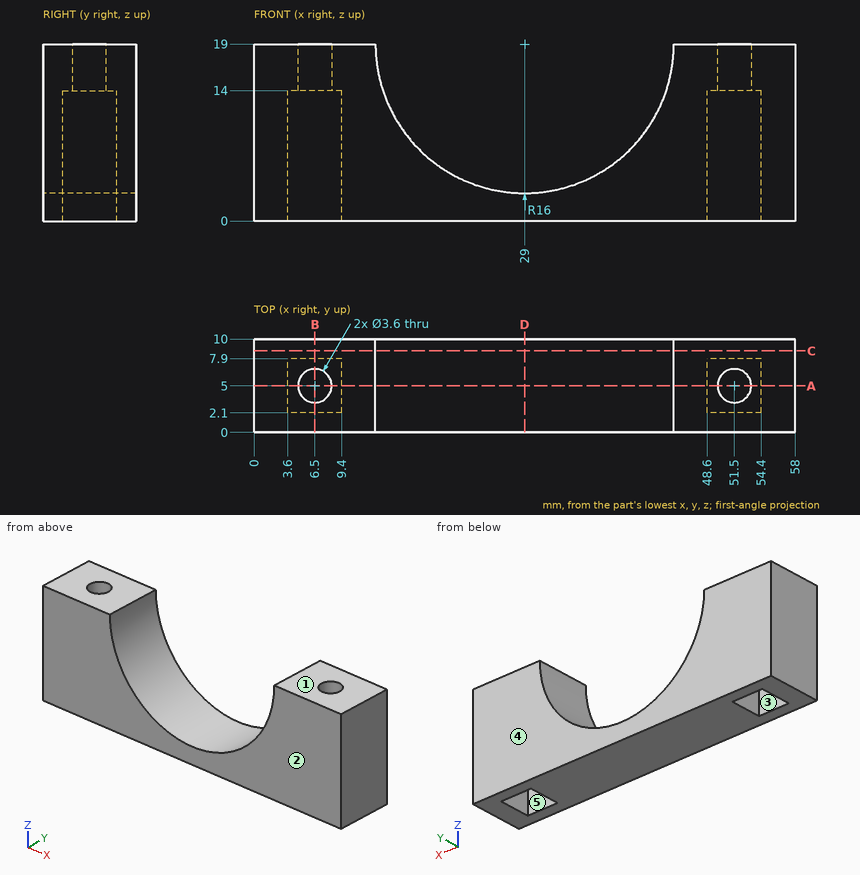
Check sheet for the drawn part. Datum: minimum x, y, z corner. Units: mm. A direction names the side the tool comes from. Coordinates: 2 decimals unless noted, no trailing zeros. Order: outer loops, then holes, each group sorted by start corner. A loop starts at its lowest first (then second) coordinate and runs counter-clockwise, first axis right, second up. Notation, with made-up numbers: M 31,10 L 73,10 A27 cw 73,36 Z; hole C 48.25,-10 d1. An arc over 180 degrees is marked long. One line per question, with ' | ' between items. Start each with the question number.
Item 1: Sectioned sample at A-A on y = 5. Record the cut outline in (x, z).
Item 2: Sectioned sample at C-C on y = 8.75. Record the cut outline in (x, z).
Item 3: Sectioned sample at B-B on x = 6.5. Record the cut outline in (y, z), and give its area (3 significant figures).
Item 4: Sectioned sample at D-D on x = 29. Record the cut outline in (y, z).
Item 5: Material ranges on line 1 (X direction, y = 5, z = 1); line 2 (Y direction, x = 6.5, z = 15); line 3 (X direction, y = 6, z = 16.5), recorded low to high.
Item 6: Gauge pin test, flat ends, axial feed: P1, Ø4, axis at x = 40, z = 14, coming from the -Y side; P2, Ø1.7, axis at x = 52.5, y = 4.5, coming from the -Z side; P3, Ø3, axis at x = 41, y = 6, coming from the +Z side. Record the tip position at first contact, or that the pin passes through.
Item 7: Mould release check, pull along Y, two halves, no side actions. Record for the marked faces 1, 2 and 3: pulls with the +Y half, pulls with the -Y half, needs draft (parallel to the pull), parting line crosses it, or undercut.
Item 8: Access from +Z, -Z, +X, -X, +Y, -Y to the whole of each face (thin tool, end or side, straight path). Record for the marked faces 4 and 5.
Answer below:
1) outline: M 0,0 L 3.6,0 L 3.6,14 L 4.7,14 L 4.7,19 L 0,19 Z; M 8.3,14 L 9.4,14 L 9.4,0 L 48.6,0 L 48.6,14 L 49.7,14 L 49.7,19 L 45,19 A16 cw 13,19 L 8.3,19 Z; M 53.3,14 L 54.4,14 L 54.4,0 L 58,0 L 58,19 L 53.3,19 Z
2) outline: M 0,0 L 58,0 L 58,19 L 45,19 A16 cw 13,19 L 0,19 Z
3) outline: M 0,0 L 2.1,0 L 2.1,14 L 3.2,14 L 3.2,19 L 0,19 Z; M 6.8,14 L 7.9,14 L 7.9,0 L 10,0 L 10,19 L 6.8,19 Z | area: 90.8 mm^2
4) outline: M 0,0 L 10,0 L 10,3 L 0,3 Z
5) line 1: x = 0 to 3.6, 9.4 to 48.6, 54.4 to 58 | line 2: y = 0 to 3.2, 6.8 to 10 | line 3: x = 0 to 5, 8 to 13.2, 44.8 to 50, 53 to 58
6) P1: passes through | P2: stops at z = 14 | P3: stops at z = 10.41
7) face 1: needs draft | face 2: pulls with the -Y half | face 3: undercut
8) face 4: +Z, -Z, +X, -X, +Y | face 5: -Z
